Work out the finished part from the listing and answer in its coordinate system (mm). Face numbers are marked on the shaded views. A direction names the side the tool comes from. Give positions to 0.01 mm unless a question says otherwise; leave off trailing zeros. Write each loop counter-clockwise with the first axis right and the second up, starting at its lowest first coordinate (ties: lowest second). Pieces come first, ordered by that corner, then holes. Notation, with made-up numbers: (81, 6) - (106, 6) arc R22 cw to (106, 21) - close; hole circle Ø6 at (48.25, 45.5). An arc over 180 degrees is marked (long way). Write item = value, one per line.
from build123d import *

# Parameters (mm, degrees)
F0_W     = 60
F0_H     = 60
F0_W_2   = 52
F0_H_2   = 52
F1_DEPTH = 170
F2_R     = 6
F3_DEPTH = 10


with BuildPart() as f1:
    # F0 (on Front) → F1 (new body)
    with BuildSketch(Plane.XZ):
        with Locations((30, 30)):
            Rectangle(F0_W, F0_H)
        with Locations((30, 30)):
            Rectangle(F0_W_2, F0_H_2, mode=Mode.SUBTRACT)
    extrude(amount=F1_DEPTH)

    # F2 (on face) → F3 (cut)
    with BuildSketch(Plane.XY.offset(60)):
        with Locations((30, -30)):
            Circle(F2_R)
    extrude(amount=-F3_DEPTH, mode=Mode.SUBTRACT)


solid = f1.part
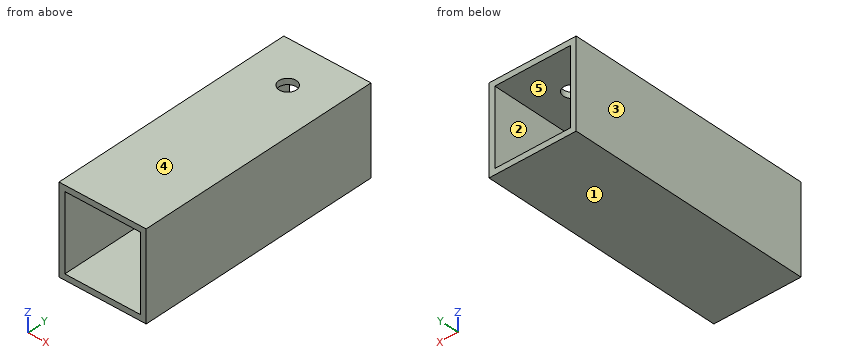
1. For a pull along Z with two mould halves and no side action, classify the marked faces 3, 4 and 5 as pulls with the +Z half, pulls with the -Z half, needs draft (parallel to the pull), parting line crosses it, or undercut.
Solution:
face_3 = needs draft
face_4 = pulls with the +Z half
face_5 = undercut
2. Given pin 1 (4 mm diameter, centred on y = -68.5, z = 33, fed in from -X); pin 2 (8 mm diameter, centred on x = 9, z = 36.5, fed in from -Y), each flat-ended and moving along its own axis, determine where each tip first touches the part or whether it passes through.
Solution:
pin_1 = 0
pin_2 = through
3. Find section C-C, the plane x = 14. Give the vertices of the cut face in (y, z), then the cut area to 3 significant figures.
Solution:
outline = (-170, 0) - (0, 0) - (0, 4) - (-170, 4) - close; (-170, 56) - (0, 56) - (0, 60) - (-170, 60) - close
area = 1,360 mm^2
4. Straight lines are drawn through the part: line 1 (Y direction, x = 30, z = 57); line 2 (Z direction, x = 28, y = -77.5). For each, find the intervals that lie inside material, in ascending order.
Solution:
line_1 = -170 to -36, -24 to 0
line_2 = 0 to 4, 56 to 60
5. Find section A-A, the plane z = 18. Give the vertices of the cut face in (x, y).
Solution:
outline = (0, -170) - (4, -170) - (4, 0) - (0, 0) - close; (56, -170) - (60, -170) - (60, 0) - (56, 0) - close
6. Find section D-D, the plane x = 30. Give the vertices of the cut face in (y, z).
Solution:
outline = (-170, 0) - (0, 0) - (0, 4) - (-170, 4) - close; (-170, 56) - (-36, 56) - (-36, 60) - (-170, 60) - close; (-24, 56) - (0, 56) - (0, 60) - (-24, 60) - close
7. A tool of negligible diameter and unlimited length cuts with its end or side. For the marked faces 1 and 2, from which of +Z, -Z, +X, -X, +Y, -Y can it reach the whole face along a straight path? Write none if from no direction.
Solution:
face_1 = -Z, +X, -X, +Y, -Y
face_2 = +Y, -Y
8. Find section B-B, the plane y = -142. Give the vertices of the cut face in (x, z).
Solution:
outline = (0, 0) - (60, 0) - (60, 60) - (0, 60) - close; hole (4, 4) - (56, 4) - (56, 56) - (4, 56) - close
